Autodesk Inventor part; units mm, degrees
ref_plane "Work Plane1" through (-24, 40, 0) normal (1, 0, 0) x (0, 1, 0)
ref_plane "XZ Plane" through (0, 0, 0) normal (0, 1, 0) x (-1, 0, 0)
ref_plane "XY Plane" through (0, 0, 0) normal (0, 0, 1) x (1, 0, 0)
sketch "Sketch3" plane through (0, 0, 0) normal (0, 0, 1) x (1, 0, 0)
  line L0 (0, 0) -> (0, 23.925) construction
  line L1 (17.75, 0) -> (17.75, 50)
  line L2 (17.75, 0) -> (19.5, 0)
  line L3 (19.5, 0) -> (19.5, 15)
  line L4 (19.5, 15) -> (24, 15)
  line L5 (24, 15) -> (24, 65)
  line L6 (17.75, 50) -> (20, 50.8189)
  line L7 (20, 50.8189) -> (20, 65)
  line L8 (20, 65) -> (24, 65)
  dimension "d9" = 35.5
  dimension "d10" = 39
  dimension "d11" = 40
  dimension "d13" = 70
  dimension "d14" = 48
  dimension "d15" = 15
  dimension "d16" = 50
  dimension "d27" = 65
revolve "Revolution2" add sketch "Sketch3" angle 360 about axis through (0, 0, 0) along (0, 1, 0)
chamfer "Chamfer1" distance 4.5 angle 45 1 edges at (-24, 15, 0)
thread "Thread1"
chamfer "Chamfer2" distance 0.5 angle 45 1 edges at (-24, 65, 0)
ref_plane "Work Plane1" through (-24, 40, 0) normal (1, 0, 0) x (0, 1, 0)
sketch "Sketch4" plane through (-24, 40, 0) normal (1, 0, 0) x (0, 1, 0)
  circle A0 centre (-5, 0) radius 2.5
  line L0 (25, 23.5) -> (25, -23.5)
  point P0 (-40, 0)
  dimension "d28" = 5
  dimension "d29" = 30
extrude "Extrusion1" cut sketch "Sketch4" along normal blind 5
thread "Thread2"
pattern_circular "Circular Pattern1" count 3 over 360 about axis through (0, 40, 0) along (0, 1, 0) of "Extrusion1"
properties part number "OringNut" material "Stainless Steel, 440C"
CAD build for the part. Positions are in the model's coordinates, mm. A direction names the side the tool comes from. Give positions to 0.01 mm unless a question says otherwise; leave off trailing zeros. Order: outer loops, then holes, each group sorted by start corner. A loop starts at its lowest first (then second) coordinate and runs counter-clockwise, first axis right, second up. Notation, with made-up numbers: (65.5, -13) - (112.5, -13) arc R24 ccw to (112.5, 14) - close; hole circle Ø1 at (16.25, -6.75). An arc over 180 degrees is marked (long way). Write each question's results on one line, items separated by ' | '.
1. Pull direction Y, two halves, no side cores. Call faces 4 (the face through (-21.54, 37.31, 0.96)), 5 (the face through (9, 0, 16)), 6 (the face through (-3.848, 25.35, 17.328)): released by +Y, released by -Y, zero draft, split by the parting line, or undercut.
Calculated:
face 4: undercut | face 5: released by -Y | face 6: zero draft
2. 3-axis set-ups, long thin cutter, end or side, ignore diameter. For faces 1 (the face through (9.53, 34.965, 16.437)), 2 (the face through (-4.336, 58.009, 19.524)), 3 (the face through (-2.539, 7.605, -19.334)): which of +Z, -Z, +X, -X, +Y, -Y reach the whole face in a straight line?
Calculated:
face 1: none | face 2: +Y | face 3: -Y
3. Probe L1, parallel to Z at x = 0, y = 11.5; L2, parallel to X at y = 58, z = 0; L3, parallel to X at y = 25, z = 0. List the from-to ranges inside material, lowest first. Write a range as from..to.
Calculated:
L1: z = -19.5..-17.75, 17.75..19.5 | L2: x = -24..-20, 20..24 | L3: x = -24..-17.75, 17.75..24
4. Saw through at C-C on y = 35. List the corners of the cut face in (x, z).
Calculated:
outline: (-23.87, -2.5) arc R24 ccw to (9.77, -21.92) - (7.33, -17.7) - (11.67, -15.2) - (14.1, -19.42) arc R24 ccw to (14.1, 19.42) - (11.67, 15.2) - (7.33, 17.7) - (9.77, 21.92) arc R24 ccw to (-23.87, 2.5) - (-19, 2.5) - (-19, -2.5) - close; hole circle Ø35.5 at (0, 0)
5. Pin check, flat tips, straight feed: pin 1 (6 mm diameter, centred on x = -4.5, y = 27, fed in from +Z); pin 2 (2 mm diameter, centred on y = 20, z = 9.5, fed in from -X); pin 3 (6 mm diameter, centred on x = 14, y = 42.5, fed in from +Z). Stop position of each tip, or through.
Calculated:
pin 1: stops at z = 23.95 | pin 2: stops at x = -22.44 | pin 3: stops at z = 21.33
